Can you work these out from the drawing? Everything is in mm from the part's minimum corner. A direction names the side the tool comes from. Give positions to 0.01 mm unless a question says otherwise; leave off trailing zeros. Write each loop counter-clockwise with the first axis right and the second up, starting at its lowest first coordinate (ties: lowest second). Pieces come first, ordered by that corner, then holes. Notation, with made-up numbers: (1, 83) -> (43, 83) arc R29 cw to (43, 108) -> close; hole circle Ø5 at (-7, 3). An arc over 180 degrees is marked (long way). Use one line per item in the form item = value.
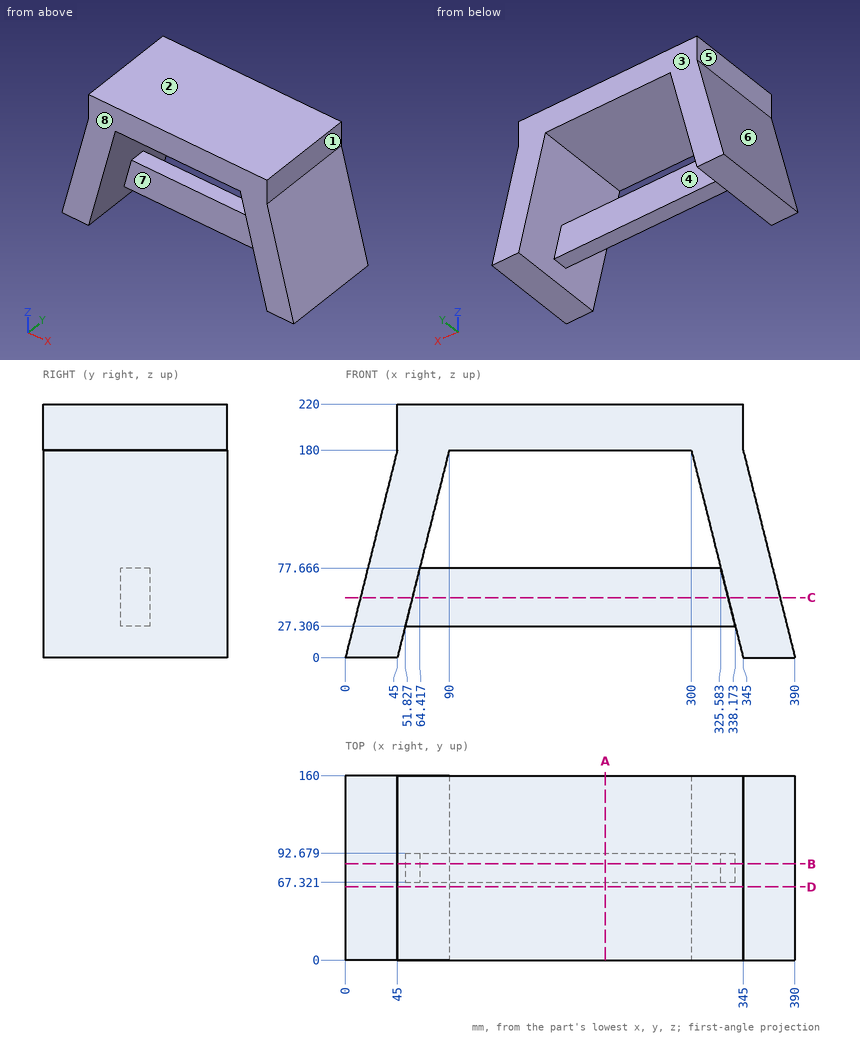
Q1. I want a section at D-D, the plane y = 63.5. Write out the boundary of the cut face in (x, z).
Result set:
outline = (0, 0) -> (45, 0) -> (90, 180) -> (300, 180) -> (345, 0) -> (390, 0) -> (345, 180) -> (345, 220) -> (45, 220) -> (45, 180) -> close
Q2. If I drill on line 1 along Z through (x, y) = (123, 77); line 2 along Z through (x, y) = (204.5, 148.5); line 3 along X through (y, z) = (123.5, 124.5) (1 decimal), over which ranges is the centre line in solid material (lowest first)? Write a range as from..to.
Result set:
line_1 = 27.31..77.67, 180..220
line_2 = 180..220
line_3 = 31.1..76.1, 313.9..358.9
Q3. I want a section at B-B, the plane y = 83.5. Write out the boundary of the cut face in (x, z).
Result set:
outline = (0, 0) -> (45, 0) -> (51.83, 27.31) -> (338.17, 27.31) -> (345, 0) -> (390, 0) -> (345, 180) -> (345, 220) -> (45, 220) -> (45, 180) -> close; hole (64.42, 77.67) -> (325.58, 77.67) -> (300, 180) -> (90, 180) -> close
Q4. If we mould it in two halves opening along X, with no side actions, what happens to the marked faces 6, 7 and 8? For each: +X half, -X half, draft (parallel to the pull), parting line (faces both ways), or undercut.
Result set:
face_6 = -X half
face_7 = undercut
face_8 = draft
Q5. Which directions (+Z, -Z, +X, -X, +Y, -Y) give clear straight access to the entire face, cutting with the end or side of a thin tool? Please do the marked faces 1, 2, 3, 4 and 5.
Result set:
face_1 = +Z, +X, +Y, -Y
face_2 = +Z, +X, -X, +Y, -Y
face_3 = +Z, -Z, +X, -X, +Y
face_4 = -Z, +Y
face_5 = +Z, -X, +Y, -Y
Q6. I want a section at A-A, the plane x = 225.5. Write out the boundary of the cut face in (y, z), and give its area (3 significant figures).
Result set:
outline = (0, 180) -> (160, 180) -> (160, 220) -> (0, 220) -> close; (67.32, 27.31) -> (92.68, 27.31) -> (92.68, 77.67) -> (67.32, 77.67) -> close
area = 7,680 mm2
Q7. I want a section at C-C, the plane z = 52. Write out the boundary of the cut face in (x, y), and give its area (3 significant figures).
Result set:
outline = (13, 0) -> (58, 0) -> (58, 67.32) -> (332, 67.32) -> (332, 0) -> (377, 0) -> (377, 160) -> (332, 160) -> (332, 92.68) -> (58, 92.68) -> (58, 160) -> (13, 160) -> close
area = 21,300 mm2
Q8. Will these pins go through, and if not, where does the flat tip stop? pin 1 Ø3 at (y, z) = (64, 132) entering from -X (1 decimal); pin 2 Ø6 at (x, y) = (222.5, 104.5) entering from -Z; pin 3 Ø8 at (x, z) = (294.5, 31) entering from +Y.
Result set:
pin_1 = 32.6
pin_2 = 180
pin_3 = 92.68
